Could you check a few things on this model? Use its own coordinates, in mm. Face numbers are marked on the shaded views. A direction names the side the tool comes from. Round coordinates to 2 decimals unless told otherwise and drop trailing zeros. Loops run counter-clockwise (first coordinate to the right, second up) from the corner with the lowest first, then second, coordinate; pieces in that order, holes last.
Autodesk Inventor part; units mm, degrees
ref_plane "YZ Plane" through (0, 0, 0) normal (1, 0, 0) x (0, 1, 0)
ref_plane "XZ Plane" through (0, 0, 0) normal (0, 1, 0) x (-1, 0, 0)
ref_plane "XY Plane" through (0, 0, 0) normal (0, 0, 1) x (1, 0, 0)
sketch "Sketch1" plane through (0, 0, 0) normal (1, 0, 0) x (0, 1, 0)
  line L0 (204.9689, 1.6371) -> (-1.9508, 1.6371)
  line L1 (-1.9508, -1.5379) -> (204.9689, -1.5379)
  circle A0 centre (-6.441, 0.0496) radius 3.175
  circle A1 centre (209.459, 0.0496) radius 3.175
  arc A2 (-1.9508, 1.6371) -> (-1.9508, -1.5379) centre (-6.441, 0.0496) ccw
  arc A3 (204.9689, -1.5379) -> (204.9689, 1.6371) centre (209.459, 0.0496) ccw
  point P0 (0, 0)
  dimension "d0" = 3.175
  dimension "d2" = 6.35
  dimension "d3" = 6.35
  dimension "d4" = 1.5875
  dimension "d5" = 1.5875
  dimension "d8" = 215.9
extrude "Extrusion1" add sketch "Sketch1" along normal blind 25.4
properties part number "aimingcontrol" material "Aluminum 6061"
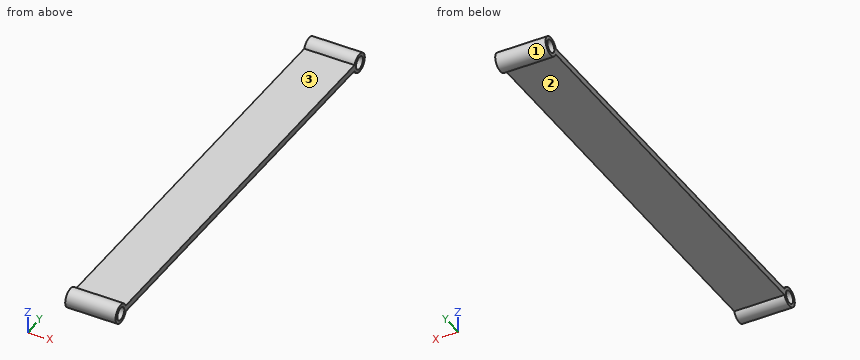
Item 1: If I drill on line 1 along Y through (x, z) = (22.5, 0.5); line 2 along Y through (x, z) = (10.5, -1); line 3 along Y through (x, z) = (23, -2.75), over which ranges is the centre line in solid material (lowest first)?
Results list:
line 1: y = -11.18 to -9.58, -3.3 to 206.32, 212.6 to 214.2
line 2: y = -11.09 to -9.44, -3.44 to 206.46, 212.46 to 214.1
line 3: y = -10.29 to -7.94, -4.94 to -2.59, 205.61 to 207.96, 210.96 to 213.31
Item 2: Will these pins go through, and if not, where does the flat tip stop? pin 1 (10 mm diameter, centred on x = 3, y = 175, fed in from +Z); pin 2 (10 mm diameter, centred on x = 12, y = 143.5, fed in from -Z).
Results list:
pin 1: stops at z = 1.64
pin 2: stops at z = -1.54
Item 3: If we section it at B-B, the plane x = 13.25: Please give me the cut outline in (y, z) (3 decimals), then the cut area to 3 significant figures.
Results list:
outline: (-1.951, -1.538) - (204.969, -1.538) arc R4.762 ccw (long way) to (204.969, 1.637) - (-1.951, 1.637) arc R4.763 ccw (long way) to start; hole circle Ø6.35 at (-6.441, 0.05); hole circle Ø6.35 at (209.459, 0.05)
area: 735 mm2
Item 4: If we section it at A-A, the plane y = 45: Please give me the cut outline in (x, z).
Results list:
outline: (0, -1.54) - (25.4, -1.54) - (25.4, 1.64) - (0, 1.64) - close
Item 5: For the marked faces 1, 2 and 3, which set-ups out of +Z, -Z, +X, -X, +Y, -Y let a thin tool reach every point of the face, with its end or its side?
Results list:
face 1: +X, -X
face 2: -Z, +X, -X
face 3: +Z, +X, -X
